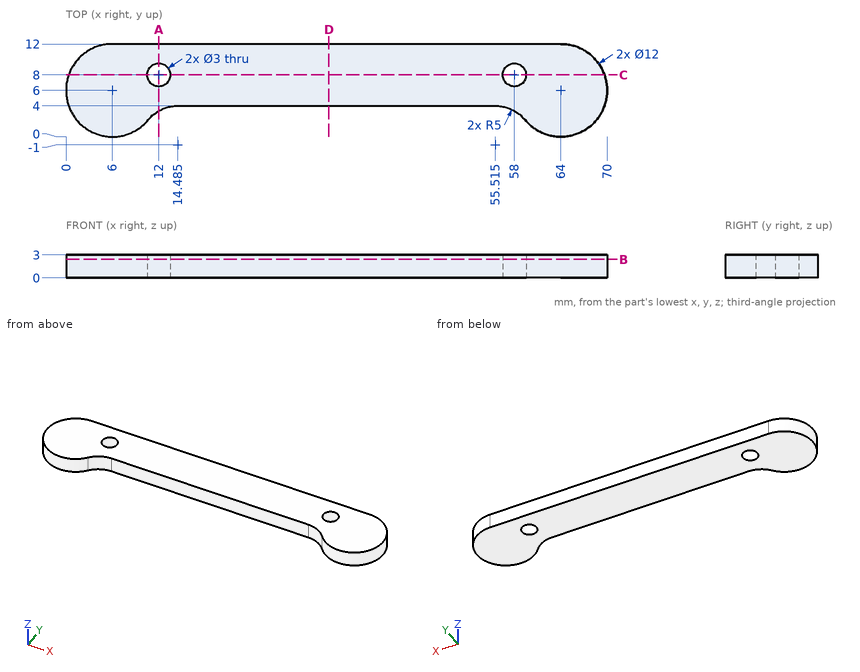
Verification items for this drawing (mm, ordinates from the low corner). Give positions to 0.01 mm unless a question says otherwise; leave off trailing zeros. Loops run counter-clockwise (first coordinate to the right, second up) from the corner with the lowest first, then second, coordinate; pieces in that order, holes last.
(1) Section check B-B on z = 2.4. Record the cut outline in (x, y) (1 decimal).
From the geometry:
outline: (6, 12) arc R6 ccw (long way) to (10.6, 2.2) arc R5 cw to (14.5, 4) - (55.5, 4) arc R5 cw to (59.4, 2.2) arc R6 ccw (long way) to (64, 12) - close; hole circle Ø3 at (12, 8); hole circle Ø3 at (58, 8)
(2) Section check A-A on x = 12. Record the cut outline in (y, z), then the cut area to 3 significant figures.
From the geometry:
outline: (3.34, 0) - (6.5, 0) - (6.5, 3) - (3.34, 3) - close; (9.5, 0) - (12, 0) - (12, 3) - (9.5, 3) - close
area: 17.0 mm2
(3) Depth check by flat-ended pin: pin 1 Ø2.5 at (x, y) = (58, 8) entering from +Z; pin 2 Ø1.5 at (y, z) = (7, 0.5) entering from -X (1 decimal). Enter the tip coordinate at first touch or a pass-through.
From the geometry:
pin 1: passes through
pin 2: stops at x = 0
(4) Section check D-D on x = 34. Record the cut outline in (y, z).
From the geometry:
outline: (4, 0) - (12, 0) - (12, 3) - (4, 3) - close
(5) Section check C-C on y = 8. Record the cut outline in (x, z), then the cut area to 3 significant figures.
From the geometry:
outline: (0.34, 0) - (10.5, 0) - (10.5, 3) - (0.34, 3) - close; (13.5, 0) - (56.5, 0) - (56.5, 3) - (13.5, 3) - close; (59.5, 0) - (69.66, 0) - (69.66, 3) - (59.5, 3) - close
area: 190 mm2
(6) Thickness scan on L1, parallel to X at y = 8, z = 1.5; L2, parallel to Y at x = 24.5, z = 1.4; L3, parallel to X at y = 2.25, z = 2.45 (1 decimal). Record the ranges inside material, lowest first.
From the geometry:
L1: x = 0.34 to 10.5, 13.5 to 56.5, 59.5 to 69.66
L2: y = 4 to 12
L3: x = 1.3 to 10.7, 59.3 to 68.7
